The listing builds one solid part. Answer for the finished solid, in the listing's coordinates (mm). Face numbers are marked on the shaded views. A direction names the side the tool comes from. Round coordinates to 2 decimals unless told otherwise and drop trailing zeros. Order: outer loops, then holes, each group sorted by start corner. A loop starts at its lowest first (then second) coordinate and runs counter-clockwise, first axis right, second up. Notation, with made-up numbers: M -2.5,49 L 24.5,49 A28 cw 24.5,81 Z; hole C -35.5,6 d8. An arc over 180 degrees is marked long. Put each result on its own line as item: value. Start each with the question number.
1. The part is cut by section A-A (y = 8.8). Count the separate pieces of the cut face and the enclosed holes in it, then the cut area to 3 significant figures.
2. Which of the six approach directions +Z, -Z, +X, -X, +Y, -Y give full straight-line access (tool end or side, diameter ignored) to the marked faces 1 and 2?
3. The part is cut by section B-B (x = -152.5). Give the vertices of the cut face in (y, z), then the cut area to 3 significant figures.
4. Consider line 1 (X direction, y = 8.8, z = -70.6); line 2 (Z direction, x = 171, y = 12.75); line 3 (Y direction, x = 145, z = -45.5). Determine where each line is inside the solid, lowest interval first.
5. This flat-tipped pin is pushed along its axis until it touches: pin 1 Ø8 at (x, z) = (-78, 35) entering from +Y. Where does it stop, or does it pass through?
6. The part is cut by section C-C (z = 29). Give the vertices of the cut face in (x, y), then the cut area to 3 significant figures.
from build123d import *

# Parameters (mm, degrees)
SKETCH_1_W                         = 400
SKETCH_1_H                         = 142
SM_BASE_FLANGE_1_DEPTH             = 0.7
SM_EDGE_FLANGE_1_STRIP_W           = 3.2
SM_EDGE_FLANGE_1_STRIP_H           = 0.7
SM_EDGE_FLANGE_1_STRIP_CUT_DEPTH   = 400
SM_EDGE_FLANGE_1_STRIP_2_W         = 3.2
SM_EDGE_FLANGE_1_STRIP_2_H         = 0.7
SM_EDGE_FLANGE_1_STRIP_CUT_2_DEPTH = 400
SM_EDGE_FLANGE_1_DEPTH             = 400
SM_EDGE_FLANGE_1_BEND_DEPTH        = 400
SKETCH_17_R                        = 3
CUT_EXTRUDE_1_DEPTH                = 10
CUT_EXTRUDE_START                  = -10
SKETCH_18_R                        = 3
CUT_EXTRUDE_2_DEPTH                = 10


# Sheet-metal steps are written as plain solids
with BuildPart() as part:
    # 草图1 → 基体-法兰1 (new body)
    with BuildSketch(Plane(origin=(0, 0, 0), x_dir=(1, 0, 0), z_dir=(0, 1, 0))):
        Rectangle(SKETCH_1_W, SKETCH_1_H)
    extrude(amount=-SM_BASE_FLANGE_1_DEPTH)

    # 边线-法兰1 strip (across the edge) → 边线-法兰1 strip cut (cut)
    with BuildSketch(Plane(origin=(200, 0, -71), x_dir=(0, 0, 1), z_dir=(-1, 0, 0))):
        with Locations((-0.7, -0.35)):
            Rectangle(SM_EDGE_FLANGE_1_STRIP_W, SM_EDGE_FLANGE_1_STRIP_H)
    extrude(amount=SM_EDGE_FLANGE_1_STRIP_CUT_DEPTH, mode=Mode.SUBTRACT)

    # 边线-法兰1 strip 2 (across the edge) → 边线-法兰1 strip cut 2 (cut)
    with BuildSketch(Plane(origin=(-200, 0, 71), x_dir=(0, 0, -1), z_dir=(1, 0, 0))):
        with Locations((-0.7, -0.35)):
            Rectangle(SM_EDGE_FLANGE_1_STRIP_2_W, SM_EDGE_FLANGE_1_STRIP_2_H)
    extrude(amount=SM_EDGE_FLANGE_1_STRIP_CUT_2_DEPTH, mode=Mode.SUBTRACT)

    # 边线-法兰1 section (across the edge) → 边线-法兰1 (add)
    with BuildSketch(Plane(origin=(200, 0, -71), x_dir=(0, 0, 1), z_dir=(-1, 0, 0))):
        with BuildLine():
            Line((0, 0.2), (0, 14.3))
            Line((0, 14.3), (0.7, 14.3))
            Line((0.7, 14.3), (0.7, 0.2))
            ThreePointArc((0.7, 0.2), (0.758578644, 0.058578644), (0.9, 0))
            Line((0.9, 0), (0.9, -0.7))
            ThreePointArc((0.9, -0.7), (0.263603897, -0.436396103), (0, 0.2))
        make_face()
    extrude(amount=SM_EDGE_FLANGE_1_DEPTH)

    # 边线-法兰1 section 2 (across the edge) → 边线-法兰1 bend (add)
    with BuildSketch(Plane(origin=(-200, 0, 71), x_dir=(0, 0, -1), z_dir=(1, 0, 0))):
        with BuildLine():
            Line((0, 0.2), (0, 14.3))
            Line((0, 14.3), (0.7, 14.3))
            Line((0.7, 14.3), (0.7, 0.2))
            ThreePointArc((0.7, 0.2), (0.758578644, 0.058578644), (0.9, 0))
            Line((0.9, 0), (0.9, -0.7))
            ThreePointArc((0.9, -0.7), (0.263603897, -0.436396103), (0, 0.2))
        make_face()
    extrude(amount=SM_EDGE_FLANGE_1_BEND_DEPTH)

    # 草图17 → 切除-拉伸1 (cut)
    with BuildSketch(Plane(origin=(0, 0, -71), x_dir=(-1, 0, 0), z_dir=(0, 0, -1))):
        with Locations(Location((-194.5, 8.8, 0), (0, 0, 90))):
            Circle(SKETCH_17_R)
        with Locations(Location((0, 8.8, 0), (0, 0, 90))):
            Circle(SKETCH_17_R)
        with Locations(Location((194.5, 8.8, 0), (0, 0, 270))):
            Circle(SKETCH_17_R)
    extrude(amount=-CUT_EXTRUDE_1_DEPTH, mode=Mode.SUBTRACT)

    # 草图18 → 切除-拉伸2 (cut)
    with BuildSketch(Plane.XY.offset(71).offset(CUT_EXTRUDE_START)):
        with Locations(Location((-194.5, 8.8, 0), (0, 0, 270))):
            Circle(SKETCH_18_R)
        with Locations(Location((0, 8.8, 0), (0, 0, 90))):
            Circle(SKETCH_18_R)
        with Locations(Location((194.5, 8.8, 0), (0, 0, 90))):
            Circle(SKETCH_18_R)
    extrude(amount=CUT_EXTRUDE_2_DEPTH, mode=Mode.SUBTRACT)


solid = part.part
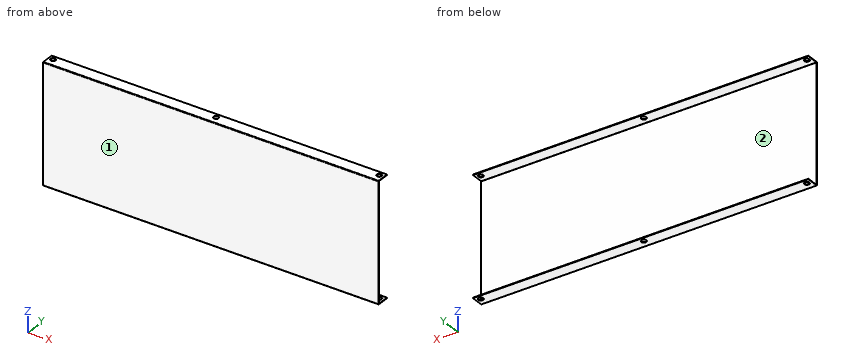
Resolved:
1. separate pieces: 8
1. enclosed holes: 0
1. area: 535 mm2
2. face 1: +Z, -Z, +X, -X, -Y
2. face 2: +X, -X, +Y
3. outline: M -0.7,-70.1 A0.9 ccw 0.2,-71 L 14.3,-71 L 14.3,-70.3 L 0.2,-70.3 A0.2 cw 0,-70.1 L 0,70.1 A0.2 cw 0.2,70.3 L 14.3,70.3 L 14.3,71 L 0.2,71 A0.9 ccw -0.7,70.1 Z
3. area: 119 mm2
4. line 1: -200 to -197.5, -191.5 to -3, 3 to 191.5, 197.5 to 200
4. line 2: -71 to -70.3, 70.3 to 71
4. line 3: -0.7 to 0
5. pin 1: y = 0
6. outline: M -200,-0.7 L 200,-0.7 L 200,0 L -200,0 Z
6. area: 280 mm2
